Autodesk Inventor part; units mm, degrees
ref_plane "IDS_WORKPLANE{1}" through (-6.35, 0, 0) normal (1, 0, 0) x (0, 0, -1)
ref_plane "Work Plane2" through (-3.175, 0, 0) normal (0, 0, -1) x (1, 0, 0)
ref_plane "YZ Plane" through (0, 0, 0) normal (1, 0, 0) x (0, 1, 0)
sketch "Sketch1" plane through (0, 0, 0) normal (0, 0, 1) x (1, 0, 0)
  line L0 (-6.35, 0) -> (88.9, 0)
  line L1 (88.9, 0) -> (88.9, 3.175)
  line L2 (88.9, 3.175) -> (0, 3.175)
  line L3 (0, 3.175) -> (0, 4.7625)
  line L4 (-27.4635, 0) -> (108.2939, 0)
  line L5 (0, -0.9525) -> (0, 5.715)
  line L6 (0, 4.7625) -> (-6.35, 4.7625)
  line L7 (-6.35, 0) -> (-6.35, 4.7625)
  arc A0 (-2.5645, 0) -> (-3.302, 2.7526) centre (-8.0696, 0) ccw
  line L8 (-6.35, 2.7526) -> (-3.302, 2.7526)
  line L9 (12.7, 3.175) -> (0, 3.175) construction
  dimension "d0" = 88.9
  dimension "d1" = 6.35
  dimension "d2" = 6.35
  dimension "d5" = 9.525
  dimension "d13" = 5.5051
  dimension "d14" = 5.5051
  dimension "d15" = 3.048
revolve "Body" add sketch "Sketch1" angle 360 about axis through (-6.35, 0, 0) along (1, 0, 0) contours A0 L8 L7 L6 L3 L5 L0 | L5 L2 L1 L0
ref_plane "IDS_WORKPLANE{1}" through (-6.35, 0, 0) normal (1, 0, 0) x (0, 0, -1)
sketch "Sketch2" plane through (-6.35, 0, 0) normal (1, 0, 0) x (0, 0, -1)
  line L0 (0, -6.6675) -> (0, 6.6675)
  line L1 (6.6675, 0) -> (-6.6675, 0)
  circle A0 centre (0, 0) radius 4.7625
  line L2 (2.6768, 0.6414) -> (2.2959, 0.6414)
  line L3 (0, 0) -> (2.6768, 0.6414) construction
  line L4 (0, 0) -> (4.0727, 3.8613) construction
  line L5 (0, 0) -> (0.783, 2.6389) construction
  line L6 (0, 0) -> (1.3763, 2.3838) construction
  line L7 (0.783, 2.6389) -> (0.5925, 2.309)
  line L8 (1.8938, 1.9975) -> (1.7034, 1.6676)
  line L9 (0, 0) -> (1.8938, 1.9975) construction
  arc A1 (2.3838, 0) -> (2.2959, 0.6414) centre (0, 0) ccw
  arc A2 (1.7034, 1.6676) -> (0.5925, 2.309) centre (0, 0) ccw
  arc A3 (2.7526, 0) -> (2.6768, 0.6414) centre (0, 0) ccw
  arc A4 (1.8938, 1.9975) -> (0.783, 2.6389) centre (0, 0) ccw
  arc A5 (2.6768, 0.6414) -> (1.6232, 2.223) centre (0, 0) ccw construction
  arc A6 (2.2959, 0.6414) -> (1.7034, 1.6676) centre (0, 0) ccw construction
  line L10 (2.6768, -0.6414) -> (2.2959, -0.6414)
  line L11 (0.783, -2.6389) -> (0.5925, -2.309)
  line L12 (1.8938, -1.9975) -> (1.7034, -1.6676)
  arc A7 (2.2959, -0.6414) -> (2.3838, 0) centre (0, 0) ccw
  arc A8 (0.5925, -2.309) -> (1.7034, -1.6676) centre (0, 0) ccw
  arc A9 (2.6768, -0.6414) -> (2.7526, 0) centre (0, 0) ccw
  arc A10 (0.783, -2.6389) -> (1.8938, -1.9975) centre (0, 0) ccw
  line L13 (-2.6768, 0.6414) -> (-2.2959, 0.6414)
  line L14 (-0.783, 2.6389) -> (-0.5925, 2.309)
  line L15 (-1.8938, 1.9975) -> (-1.7034, 1.6676)
  arc A11 (-2.2959, 0.6414) -> (-2.3838, 0) centre (0, 0) ccw
  arc A12 (-0.5925, 2.309) -> (-1.7034, 1.6676) centre (0, 0) ccw
  arc A13 (-2.6768, 0.6414) -> (-2.7526, 0) centre (0, 0) ccw
  arc A14 (-0.783, 2.6389) -> (-1.8938, 1.9975) centre (0, 0) ccw
  line L16 (-0.783, -2.6389) -> (-0.5925, -2.309)
  arc A15 (-1.7034, -1.6676) -> (-0.5925, -2.309) centre (0, 0) ccw
  line L17 (-1.8938, -1.9975) -> (-1.7034, -1.6676)
  arc A16 (-1.8938, -1.9975) -> (-0.783, -2.6389) centre (0, 0) ccw
  arc A17 (-2.3838, 0) -> (-2.2959, -0.6414) centre (0, 0) ccw
  line L18 (-2.6768, -0.6414) -> (-2.2959, -0.6414)
  arc A18 (-2.7526, 0) -> (-2.6768, -0.6414) centre (0, 0) ccw
  point P0 (1.3763, -2.3838)
  point P1 (-1.3763, 2.3838)
  point P2 (-1.3763, -2.3838)
  dimension "d19" = 0.6413
  dimension "d20" = 1.2827
  dimension "d21" = 33.052
  dimension "d22" = 5.5051
  dimension "d23" = 4.7676
extrude "Slot" add sketch "Sketch2" along normal up to next contours A1 L2 A3 L1 | L1 A9 L10 A7 | A17 L18 A18 L1 | L1 A13 L13 A11 | A4 L8 A2 L7 | L11 A8 L12 A10 | L14 A12 L15 A14 | A16 L17 A15 L16
fillet "Fillet1" radius 0.635 1 edges at (-6.35, -4.7625, 0)
thread "Thread"
chamfer "Chamfer1" distance 0.7556 distance2 0.7556 1 edges at (88.9, -3.175, 0) measured on face at (88.9, 1.0276, 0.2533)
ref_plane "Work Plane2" through (-3.175, 0, 0) normal (0, 0, -1) x (1, 0, 0)
equation "\"d19\" = 0.5 * SBR"
equation "\"d20\" = SBR"
equation "\"d22\" = 1.1547 * SW"
equation "\"d23\" = SW"
equation "\"d17\" = INTI"
equation "\"d24\" = RR"
equation "\"d6\" = GEL"
equation "\"d9\" = -0.5 * SPD + 0.5 * NND"
equation "\"d10\" = GUL"
equation "\"d0\" = NLG"
equation "\"d1\" = KOH"
equation "\"d2\" = NND"
equation "\"d5\" = KOD"
equation "\"d13\" = 1.1547 * SW"
equation "\"d14\" = 1.1547 * SW"
equation "\"d15\" = INTI"
equation "\"NND\" = 6.35"
equation "\"NLG\" = 88.9"
equation "\"GEL\" = 25.4"
equation "\"KOD\" = 9.525"
equation "\"KOH\" = 6.35"
equation "\"SPD\" = GD1"
equation "\"GUL\" = 0.75565"
equation "\"SBR\" = 1.2827"
equation "\"INTI\" = 3.048"
equation "\"d11\" = -KOH"
equation "\"SW\" = 4.76758"
equation "\"d16\" = 1.1547 * SW"
equation "\"d18\" = SW"
equation "\"RR\" = 0.635"
equation "\"TOA\" = 30deg"
equation "\"GD1\" = 4.8387"
equation "\"THREADDIA\" = 6.35"
equation "\"BDM\" = NND"
equation "\"GD\" = NND"
equation "\"GAL\" = 3.175"
equation "\"E0\" = 5.55498"
properties part number "ANSI B18.3 - 1/4-20 UNC - 3.5" material "Steel, Mild"
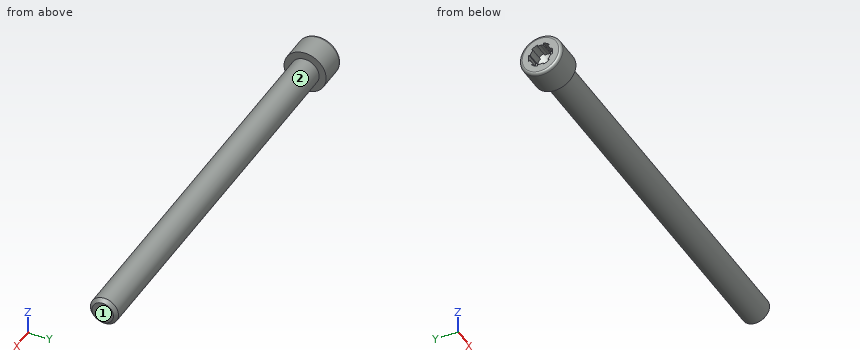
Verification items for the finished model (mm, model axes). Face numbers are marked on the shaded views. A direction names the side the tool comes from. Coordinates: 2 decimals unless noted, no trailing zeros. Order: outer loops, then holes, each group sorted by start corner. A loop starts at its lowest first (then second) coordinate and runs counter-clockwise, first axis right, second up.
Item 1: Material ranges on L1, parallel to X at y = 0, z = -0.25; L2, parallel to X at y = 3.25, z = 0.25; L3, parallel to Z at x = 74, y = 0 (3 decimals), recorded low to high.
Filled in:
L1: x = -2.57 to 88.9
L2: x = -6.35 to 0
L3: z = -3.175 to 3.175
Item 2: Depth check by flat-ended pin: pin 1 (1 mm diameter, centred on x = 77, z = -2, fed in from -Y); pin 2 (1.5 mm diameter, centred on x = 69.5, y = -2.5, fed in from -Z); pin 3 (4 mm diameter, centred on x = 49.5, y = 3.5, fed in from +Z). Enter the tip coordinate at first touch or a pass-through.
Filled in:
pin 1: stops at y = -2.8
pin 2: stops at z = -2.65
pin 3: stops at z = 2.8
Item 3: Access from +Z, -Z, +X, -X, +Y, -Y to the whole of each face (thin tool, end or side, straight path). Record for the marked faces 1 and 2.
Filled in:
face 1: +Z, -Z, +X, +Y, -Y
face 2: +X
Item 4: Section check A-A, the plane x = 7. Enter the section's corners in (y, z) (3 decimals), then the cut area to 3 significant figures.
Filled in:
outline: circle Ø6.35 at (0, 0)
area: 31.7 mm2
